from build123d import *

# Parameters (mm, degrees)
SKETCH1_R           = 8.5
BOSS_EXTRUDE1_DEPTH = 0.6


with BuildPart() as part:
    # Sketch1 → Boss-Extrude1 (new body)
    with BuildSketch(Plane(origin=(0, 0, 0), x_dir=(1, 0, 0), z_dir=(0, 1, 0))):
        with BuildLine():
            Line((-0.5, -14.241225369), (-0.5, -13.75))
            ThreePointArc((-0.5, -13.75), (0, -13.25), (0.5, -13.75))
            Line((0.5, -13.75), (0.5, -14.241225369))
            ThreePointArc((0.5, -14.241225369), (5.453238911, -13.165283338), (9.71651364, -10.423620421))
            Line((9.71651364, -10.423620421), (9.369164851, -10.076271632))
            ThreePointArc((9.369164851, -10.076271632), (9.369164851, -9.369164851), (10.076271632, -9.369164851))
            Line((10.076271632, -9.369164851), (10.423620421, -9.71651364))
            ThreePointArc((10.423620421, -9.71651364), (13.165283338, -5.453238911), (14.241225369, -0.5))
            Line((14.241225369, -0.5), (13.75, -0.5))
            ThreePointArc((13.75, -0.5), (13.25, 0), (13.75, 0.5))
            Line((13.75, 0.5), (14.241225369, 0.5))
            ThreePointArc((14.241225369, 0.5), (13.165283338, 5.453238911), (10.423620421, 9.71651364))
            Line((10.423620421, 9.71651364), (10.076271632, 9.369164851))
            ThreePointArc((10.076271632, 9.369164851), (9.369164851, 9.369164851), (9.369164851, 10.076271632))
            Line((9.369164851, 10.076271632), (9.71651364, 10.423620421))
            ThreePointArc((9.71651364, 10.423620421), (5.453238911, 13.165283338), (0.5, 14.241225369))
            Line((0.5, 14.241225369), (0.5, 13.75))
            ThreePointArc((0.5, 13.75), (0, 13.25), (-0.5, 13.75))
            Line((-0.5, 13.75), (-0.5, 14.241225369))
            ThreePointArc((-0.5, 14.241225369), (-5.453238911, 13.165283338), (-9.71651364, 10.423620421))
            Line((-9.71651364, 10.423620421), (-9.369164851, 10.076271632))
            ThreePointArc((-9.369164851, 10.076271632), (-9.369164851, 9.369164851), (-10.076271632, 9.369164851))
            Line((-10.076271632, 9.369164851), (-10.423620421, 9.71651364))
            ThreePointArc((-10.423620421, 9.71651364), (-13.165283338, 5.453238911), (-14.241225369, 0.5))
            Line((-14.241225369, 0.5), (-13.75, 0.5))
            ThreePointArc((-13.75, 0.5), (-13.25, 0), (-13.75, -0.5))
            Line((-13.75, -0.5), (-14.241225369, -0.5))
            ThreePointArc((-14.241225369, -0.5), (-13.165283338, -5.453238911), (-10.423620421, -9.71651364))
            Line((-10.423620421, -9.71651364), (-10.076271632, -9.369164851))
            ThreePointArc((-10.076271632, -9.369164851), (-9.369164851, -9.369164851), (-9.369164851, -10.076271632))
            Line((-9.369164851, -10.076271632), (-9.71651364, -10.423620421))
            ThreePointArc((-9.71651364, -10.423620421), (-5.453238911, -13.165283338), (-0.5, -14.241225369))
        make_face()
        with BuildLine():
            Line((-9.4, 3), (-9.4, -3))
            ThreePointArc((-9.4, -3), (-10, -3.6), (-10.6, -3))
            Line((-10.6, -3), (-10.6, 3))
            ThreePointArc((-10.6, 3), (-10, 3.6), (-9.4, 3))
        make_face(mode=Mode.SUBTRACT)
        with Locations(Location((0, 0, 0), (0, 0, 270))):
            Circle(SKETCH1_R, mode=Mode.SUBTRACT)
        with BuildLine():
            ThreePointArc((10.6, -3), (10, -3.6), (9.4, -3))
            Line((9.4, -3), (9.4, 3))
            ThreePointArc((9.4, 3), (10, 3.6), (10.6, 3))
            Line((10.6, 3), (10.6, -3))
        make_face(mode=Mode.SUBTRACT)
    extrude(amount=BOSS_EXTRUDE1_DEPTH)


solid = part.part
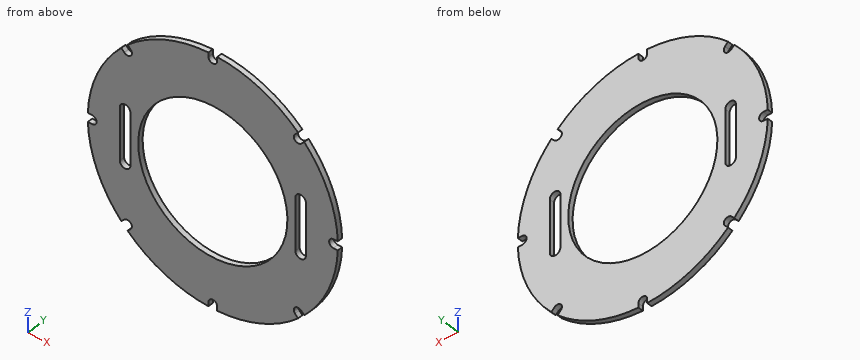
Input: part model. Units: mm. Frame: model coordinates. Round coordinates to 2 decimals unless told otherwise and drop trailing zeros. Loops run counter-clockwise (first coordinate to the right, second up) from the corner with the lowest first, then second, coordinate; pieces in that order, holes last. Notation, with made-up numbers: M 37.5,39.25 L 93.5,39.25 A20 ccw 93.5,73.25 Z; hole C 43.25,1 d9. An arc over 180 degrees is marked long. Answer as CSV lines item,"result". Start each with the question number.
(1) Section B-B, the plane z = -7. Output: boundary loops of the cut face in (x, y), plus the area to 3 significant figures.
(2) Section D-D, the plane x = -11. Output: boundary loops of the cut face in (y, z).
(3) Section C-C, the plane y = 0.5. State how many separate pieces and enclosed holes the cut face has, plus the area to 3 significant figures.
(4) Section A-A, the plane x = -1.5. Output: boundary loops of the cut face in (y, z).
(5) Line query: line 1 (X direction, y = 0.1, z = 0); line 2 (X direction, y = 0.4, z = -5.75); line 3 (Z direction, x = -2.5, y = 0.3). Output: solid intervals per line, ascending. Write a range as [from, to].
Values found:
1,outline,"M -12.41,0 L -4.82,0 L -4.82,0.6 L -12.41,0.6 Z; M 4.82,0 L 12.41,0 L 12.41,0.6 L 4.82,0.6 Z"
1,area,"9.11 mm²"
2,outline,"M 0,-9.06 L 0.6,-9.06 L 0.6,9.06 L 0,9.06 Z"
3,separate pieces,"1"
3,enclosed holes,"3"
3,area,"387 mm²"
4,outline,"M 0,-14.17 L 0.6,-14.17 L 0.6,-8.37 L 0,-8.37 Z; M 0,8.37 L 0.6,8.37 L 0.6,14.17 L 0,14.17 Z"
5,line 1,"x = [-13.25, -10.6], [-9.4, -8.5], [8.5, 9.4], [10.6, 13.25]"
5,line 2,"x = [-13.04, -6.26], [6.26, 13.04]"
5,line 3,"z = [-14.03, -8.12], [8.12, 14.03]"
